Geometry: see drawing. Coordinates: mm, zero at the bounding-box minimum. Give positions to 0.01 mm unless a question says otherwise; leave off trailing zeros. Write each loop counter-clockwise with the first axis right and the second up, starting at its lowest first coordinate (ties: lowest second). Pieces come first, ordered by that corner, then holes. Notation, with made-up numbers: (63.5, 42) - (92.5, 42) arc R24 ccw to (92.5, 74) - close; hole circle Ø4 at (30.5, -5). An arc over 180 degrees is marked (long way). Use CSV: the item, a comma, the result in double quotes. Start each with the question number.
(1) Section D-D on x = 80.5. Output: boundary loops of the cut face in (y, z).
(2) Line query: probe 1 along X at (y, z) = (3.65, 50.8); probe 2 along X at (y, z) = (2.5, 62.5); probe 3 along Z at (x, y) = (26.5, 3.9). Output: solid intervals per line, ascending. Write a range as [from, to].
(3) Section C-C on z = 86.5. Output: boundary loops of the cut face in (x, y).
(4) Section B-B on x = 31.5. Output: boundary loops of the cut face in (y, z), and give its area (3 significant figures).
(5) First-contact query: pin 1 Ø3 at (y, z) = (2.5, 2) entering from +X; pin 2 Ø1.8 at (y, z) = (2.5, 56.5) entering from -X; pin 3 Ø10 at (x, z) = (92, 17) entering from -Y; pin 4 Ø3 at (x, y) = (2, 4) entering from -Z. Flat tips, straight axial feed; report the tip coordinate or a pass-through.
(6) Section A-A on z = 50.8. Output: boundary loops of the cut face in (x, y).
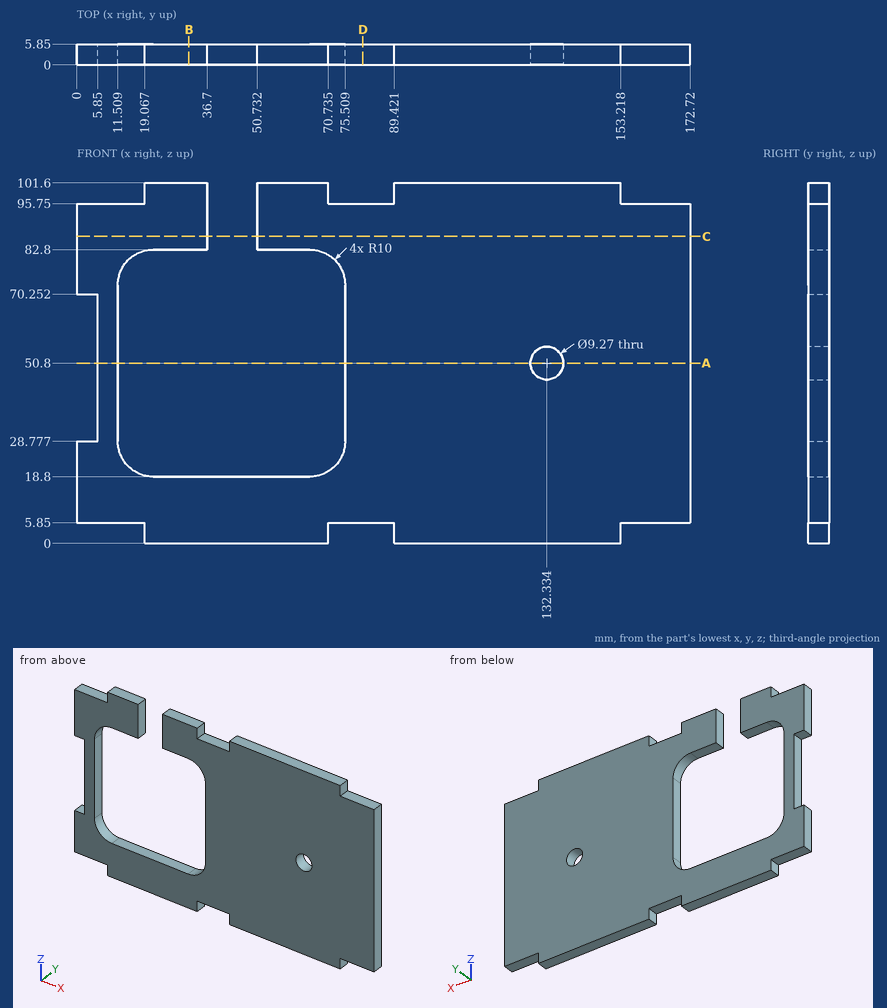
Check values:
1,outline,"(0, 5.85) - (5.85, 5.85) - (5.85, 95.75) - (0, 95.75) - close"
2,probe 1,"x = [5.85, 11.51], [75.51, 127.7], [136.97, 172.72]"
2,probe 2,"x = [5.85, 11.51], [75.51, 172.72]"
2,probe 3,"z = [0, 18.8], [82.8, 101.6]"
3,outline,"(0, 0) - (36.7, 0) - (36.7, 5.85) - (0, 5.85) - close; (50.73, 0) - (172.72, 0) - (172.72, 5.85) - (50.73, 5.85) - close"
4,outline,"(0, 0) - (5.85, 0) - (5.85, 18.8) - (0, 18.8) - close; (0, 82.8) - (5.85, 82.8) - (5.85, 101.6) - (0, 101.6) - close"
4,area,"220 mm²"
5,pin 1,"stops at x = 153.22"
5,pin 2,"stops at x = 5.85"
5,pin 3,"stops at y = 0"
5,pin 4,"stops at z = 5.85"
6,outline,"(5.85, 0) - (11.51, 0) - (11.51, 5.85) - (5.85, 5.85) - close; (75.51, 0) - (127.7, 0) - (127.7, 5.85) - (75.51, 5.85) - close; (136.97, 0) - (172.72, 0) - (172.72, 5.85) - (136.97, 5.85) - close"
